```python
from build123d import *

# Parameters (mm, degrees)
SKETCH1_W                     = 80
SKETCH1_H                     = 105
BOSS_EXTRUDE1_DEPTH           = 20
CUT_EXTRUDE4_DEPTH            = 20
CUT_EXTRUDE4_DEPTH_BACK       = 20
SKETCH1_3_R                   = 3
SKETCH1_3_R_2                 = 1.5
SKETCH2_W                     = 76
SKETCH2_H                     = 101
CUT_EXTRUDE5_DEPTH            = 18
SKETCH3_R                     = 6.5
CUT_EXTRUDE6_DEPTH            = 18
SKETCH5_R                     = 8.5
BOSS_EXTRUDE2_DEPTH           = 4
BOSS_EXTRUDE3_START           = 4
SKETCH6_R                     = 8.5
BOSS_EXTRUDE3_DEPTH           = 4
SKETCH7_R                     = 7
CUT_EXTRUDE7_DEPTH            = 24
SKETCH8_W                     = 30
SKETCH8_H                     = 1.5
BOSS_EXTRUDE4_DEPTH           = 14
SKETCH9_R                     = 2.5
CUT_EXTRUDE8_DEPTH            = 14
SKETCH10_W                    = 21
SKETCH10_H                    = 15
CUT_EXTRUDE9_DEPTH            = 14
FILLET1_R                     = 2
SKETCH11_R                    = 3
BOSS_EXTRUDE5_DEPTH           = 20
TAP_DRILL_FOR_4_40_TAP2_D     = 2.2606
TAP_DRILL_FOR_4_40_TAP2_DEPTH = 13.05
TAP_DRILL_FOR_4_40_TAP2_TIP   = 0.679152758


with BuildPart() as part:
    # Sketch1 → Boss-Extrude1 (new body)
    with BuildSketch(Plane.XY):
        with Locations((1071.513868959, -1418.75124805)):
            Rectangle(SKETCH1_W, SKETCH1_H)
    extrude(amount=BOSS_EXTRUDE1_DEPTH)

    # Sketch1_3 → Cut-Extrude4 (cut, two sides: drawn at the far end of the back side and taken through both)
    with BuildSketch(Plane.XY.offset(-CUT_EXTRUDE4_DEPTH_BACK)):
        with Locations((1087.513868959, -1418.25124805)):
            Circle(SKETCH1_3_R)
        with Locations((1087.513868959, -1405.75124805)):
            Circle(SKETCH1_3_R_2)
        with Locations((1070.013868959, -1405.75124805)):
            Circle(SKETCH1_3_R_2)
        with Locations((1070.013868959, -1418.25124805)):
            Circle(SKETCH1_3_R)
    extrude(amount=CUT_EXTRUDE4_DEPTH + CUT_EXTRUDE4_DEPTH_BACK, mode=Mode.SUBTRACT)

    # Sketch2 → Cut-Extrude5 (cut)
    with BuildSketch(Plane(origin=(0, 0, 0), x_dir=(-1, 0, 0), z_dir=(0, 0, -1))):
        with Locations((-1071.513868959, -1418.75124805)):
            Rectangle(SKETCH2_W, SKETCH2_H)
    extrude(amount=-CUT_EXTRUDE5_DEPTH, mode=Mode.SUBTRACT)

    # Sketch3 → Cut-Extrude6 (cut)
    with BuildSketch(Plane.ZY.offset(-1109.513868959)):
        with Locations((9, -1380.25124805)):
            Circle(SKETCH3_R)
    extrude(amount=-CUT_EXTRUDE6_DEPTH, mode=Mode.SUBTRACT)

    # Sketch5 → Boss-Extrude2 (add)
    with BuildSketch(Plane(origin=(1111.513868959, 0, 0), x_dir=(0, 0, -1), z_dir=(1, 0, 0))):
        with Locations(Location((-9, -1380.25124805, 0), (0, 0, 90))):
            Circle(SKETCH5_R)
    extrude(amount=BOSS_EXTRUDE2_DEPTH)

    # Sketch6 → Boss-Extrude3 (add)
    with BuildSketch(Plane.ZY.offset(-1109.513868959).offset(BOSS_EXTRUDE3_START)):
        with Locations(Location((9, -1380.25124805, 0), (0, 0, 90))):
            Circle(SKETCH6_R)
    extrude(amount=-BOSS_EXTRUDE3_DEPTH)

    # Sketch7 → Cut-Extrude7 (cut)
    with BuildSketch(Plane(origin=(1115.513868959, 0, 0), x_dir=(0, 0, -1), z_dir=(1, 0, 0))):
        with Locations(Location((-9, -1380.25124805, 0), (0, 0, 90))):
            Circle(SKETCH7_R)
    extrude(amount=-CUT_EXTRUDE7_DEPTH, mode=Mode.SUBTRACT)

    # Sketch8 → Boss-Extrude4 (add)
    with BuildSketch(Plane(origin=(0, 0, 18), x_dir=(-1, 0, 0), z_dir=(0, 0, -1))):
        with Locations((-1087.013868959, -1389.00124805)):
            Rectangle(SKETCH8_W, SKETCH8_H)
    extrude(amount=BOSS_EXTRUDE4_DEPTH)

    # Sketch9 → Cut-Extrude8 (cut)
    with BuildSketch(Plane(origin=(0, -1469.25124805, 0), x_dir=(1, 0, 0), z_dir=(0, 1, 0))):
        with Locations((1071.513868959, 0)):
            Circle(SKETCH9_R)
    extrude(amount=-CUT_EXTRUDE8_DEPTH, mode=Mode.SUBTRACT)

    # Sketch10 → Cut-Extrude9 (cut)
    with BuildSketch(Plane(origin=(0, -1366.25124805, 0), x_dir=(1, 0, 0), z_dir=(0, 1, 0))):
        with Locations((1048.013868959, -9.5)):
            Rectangle(SKETCH10_W, SKETCH10_H)
    extrude(amount=-CUT_EXTRUDE9_DEPTH, mode=Mode.SUBTRACT)

    # Fillet1
    fillet1_edges = [part.edges().sort_by_distance(p)[0] for p in [
        (1111.513868959, -1418.75124805, 20),
        (1071.513868959, -1366.25124805, 20),
        (1031.513868959, -1418.75124805, 20),
        (1071.513868959, -1471.25124805, 20),
    ]]
    fillet(fillet1_edges, radius=FILLET1_R)

    # Sketch11 → Boss-Extrude5 (add)
    with BuildSketch(Plane(origin=(0, 0, 18), x_dir=(-1, 0, 0), z_dir=(0, 0, -1))):
        with Locations((-1039.513868959, -1419.25124805)):
            Circle(SKETCH11_R)
    extrude(amount=BOSS_EXTRUDE5_DEPTH)

    # Tap Drill for _4-40 Tap2
    with Locations(Plane(origin=(0, 0, -2), x_dir=(-1, 0, 0), z_dir=(0, 0, -1))):
        with Locations((-1039.426320133, -1419.282531473)):
            Hole(TAP_DRILL_FOR_4_40_TAP2_D / 2, depth=TAP_DRILL_FOR_4_40_TAP2_DEPTH)
            with Locations((0, 0, -(TAP_DRILL_FOR_4_40_TAP2_DEPTH + TAP_DRILL_FOR_4_40_TAP2_TIP / 2))):  # 118° drill point
                Cone(0, TAP_DRILL_FOR_4_40_TAP2_D / 2, TAP_DRILL_FOR_4_40_TAP2_TIP, mode=Mode.SUBTRACT)


solid = part.part
```
The listing builds one solid part. Answer for the finished solid, in the listing's coordinates (mm). A direction names the side the tool comes from. Coordinates: 2 decimals unless noted, no trailing zeros. Write each loop counter-clockwise with the first axis right and the second up, starting at its lowest first coordinate (ties: lowest second). Pieces come first, ordered by that corner, then holes. Notation, with made-up numbers: (14, 84) -> (62, 84) arc R5 cw to (62, 90) -> close; hole circle Ø11 at (47.25, -7.75). An arc over 180 degrees is marked (long way). Write each question's results on one line, items separated by ' | '. Start each with the question number.
1) A cutting plane is placed at B-B (z = 13.75). Count the separate pieces of the cut face and the enclosed holes in it, then the cut area to 3 significant figures.
2) A cutting plane is placed at D-D (x = 1082). Determine the outline of the cut face in (y, z), then the cut area to 3 significant figures.
3) Flat-ended cylindrical pins translate along their axes: pin 1 Ø1.5 at (y, z) = (-1437, 8) entering from +X; pin 2 Ø2 at (x, y) = (1048, -1367.5) entering from -Z; pin 3 Ø4 at (y, z) = (-1383, 7.5) entering from +X. Find the tip coordinate at first contact, or state that the pin passes through.
4) For a pull along X with two mould halves and no side action, classify faces 5 (the cylindrical face through (1086.408, -1404.737, 18.986)), 6 (the cylindrical face through (1068.908, -1404.737, 18.986)), 7 (the flat face through (1071, -1368, 0)), 8 (the flat face through (1115.514, -1378, 16)) as +X half, -X half, draft (parallel to the pull), parting line (faces both ways), or undercut.
5) A tool of negligible diameter and unlimited length cuts with its end or side. For faces 1 (the cylindrical face through (1107.486, -1372.144, 6.447)), 2 (the cylindrical face through (1040.47, -1419.72, 4.62)), 3 (the cylindrical face through (1071.5, -1470.2, 2.5)), 4 (the cylindrical face through (1110.584, -1373.785, 6.319)), from which of +Z, -Z, +X, -X, +Y, -Y can it reach the whole face along a straight path? Write none if from no direction.
6) A cutting plane is placed at A-A (x = 1053). Determine the outline of the cut face in (y, z).
7) Straight lines are drawn through the part: probe 1 along X at (y, z) = (-1419, 16); probe 2 along Y at (x, z) = (1091.5, 12.75); probe 3 along Y at (x, z) = (1055, 17.5). For each, find the intervals that lie inside material, in ascending order.
8) A cutting plane is placed at C-C (y = -1454). Determine the outline of the cut face in (x, z), then the cut area to 3 significant figures.
Values follow:
1) separate pieces: 4 | enclosed holes: 0 | area: 765 mm²
2) outline: (-1471.25, 0) -> (-1469.25, 0) -> (-1469.25, 18) -> (-1389.75, 18) -> (-1389.75, 4) -> (-1388.25, 4) -> (-1388.25, 18) -> (-1368.25, 18) -> (-1368.25, 0) -> (-1366.25, 0) -> (-1366.25, 18) arc R2 ccw to (-1368.25, 20) -> (-1469.25, 20) arc R2 ccw to (-1471.25, 18) -> close | area: 301 mm²
3) pin 1: x = 1111.51 | pin 2: z = 0 | pin 3: x = 1033.51
4) face 5: undercut | face 6: undercut | face 7: draft | face 8: +X half
5) face 1: none | face 2: -Z | face 3: -Z, -Y | face 4: +X
6) outline: (-1471.25, 0) -> (-1469.25, 0) -> (-1469.25, 18) -> (-1368.25, 18) -> (-1368.25, 17) -> (-1366.25, 17) -> (-1366.25, 18) arc R2 ccw to (-1368.25, 20) -> (-1469.25, 20) arc R2 ccw to (-1471.25, 18) -> close; (-1368.25, 0) -> (-1366.25, 0) -> (-1366.25, 2) -> (-1368.25, 2) -> close
7) probe 1: 1031.51 to 1033.51, 1036.52 to 1042.5, 1109.51 to 1111.51 | probe 2: -1471.25 to -1469.25, -1389.75 to -1388.25, -1368.25 to -1366.25 | probe 3: -1471.25 to -1469.25, -1368.25 to -1366.25
8) outline: (1031.51, 0) -> (1033.51, 0) -> (1033.51, 18) -> (1109.51, 18) -> (1109.51, 0) -> (1111.51, 0) -> (1111.51, 18) arc R2 ccw to (1109.51, 20) -> (1033.51, 20) arc R2 ccw to (1031.51, 18) -> close | area: 230 mm²
